```python
from build123d import *

# Parameters (mm, degrees)
SKETCH1_W           = 30
SKETCH1_H           = 12.2
BOSS_EXTRUDE1_DEPTH = 30
SKETCH2_W           = 26
SKETCH2_H           = 4.3
CUT_EXTRUDE1_DEPTH  = 26
SKETCH3_W           = 30
SKETCH3_H           = 30
BOSS_EXTRUDE2_DEPTH = 26
SKETCH4_W           = 17.8
SKETCH4_H           = 17.78
CUT_EXTRUDE2_DEPTH  = 26
SKETCH6_W           = 4.42
SKETCH6_H           = 26
CUT_EXTRUDE3_DEPTH  = 17.8
SKETCH9_W           = 4.3
SKETCH9_H           = 26
CUT_EXTRUDE4_DEPTH  = 17.8


with BuildPart() as part:
    # Sketch1 → Boss-Extrude1 (new body)
    with BuildSketch(Plane.XY):
        with Locations((-26.249929658, 18.197752809)):
            Rectangle(SKETCH1_W, SKETCH1_H)
    extrude(amount=BOSS_EXTRUDE1_DEPTH)

    # Sketch2 → Cut-Extrude1 (cut)
    with BuildSketch(Plane(origin=(-11.249929658, 0, 0), x_dir=(0, 0, -1), z_dir=(1, 0, 0))):
        with Locations((-17, 18.197752809)):
            Rectangle(SKETCH2_W, SKETCH2_H)
    extrude(amount=-CUT_EXTRUDE1_DEPTH, mode=Mode.SUBTRACT)

    # Sketch3 → Boss-Extrude2 (add)
    with BuildSketch(Plane(origin=(0, 24.297752809, 0), x_dir=(1, 0, 0), z_dir=(0, 1, 0))):
        with Locations((-26.249929658, -15)):
            Rectangle(SKETCH3_W, SKETCH3_H)
    extrude(amount=BOSS_EXTRUDE2_DEPTH)

    # Sketch4 → Cut-Extrude2 (cut)
    with BuildSketch(Plane(origin=(0, 50.297752809, 0), x_dir=(1, 0, 0), z_dir=(0, 1, 0))):
        with Locations((-20.149929658, -21.11)):
            Rectangle(SKETCH4_W, SKETCH4_H)
    extrude(amount=-CUT_EXTRUDE2_DEPTH, mode=Mode.SUBTRACT)

    # Sketch6 → Cut-Extrude3 (cut)
    with BuildSketch(Plane(origin=(-11.249929658, 0, 0), x_dir=(0, 0, -1), z_dir=(1, 0, 0))):
        with Locations((-6.11, 37.297752809)):
            Rectangle(SKETCH6_W, SKETCH6_H)
    extrude(amount=-CUT_EXTRUDE3_DEPTH, mode=Mode.SUBTRACT)

    # Sketch9 → Cut-Extrude4 (cut)
    with BuildSketch(Plane.XY.offset(30)):
        with Locations((-35.149929658, 37.297752809)):
            Rectangle(SKETCH9_W, SKETCH9_H)
    extrude(amount=-CUT_EXTRUDE4_DEPTH, mode=Mode.SUBTRACT)


solid = part.part
```
Here's how the part is built. I have some questions about the finished solid (model axes, mm). A direction names the side the tool comes from. Coordinates: 2 decimals unless noted, no trailing zeros. Write each loop counter-clockwise with the first axis right and the second up, starting at its lowest first coordinate (ties: lowest second). Pieces come first, ordered by that corner, then holes. Notation, with made-up numbers: M 16.5,-38 L 55.5,-38 A27 cw 55.5,-11 Z; hole C 4.25,-4.5 d5. An arc over 180 degrees is marked long. Answer as CSV lines item,"result". Start each with the question number.
Q1. Suppose I cut it at A-A, the plane z = 9.5. List the corners of the cut face in (x, y) for me, then the cut area to 3 significant figures.
Q2. Will these pins go through, and if not, where does the flat tip stop? pin 1 Ø3.5 at (y, z) = (18.5, 23) entering from +X; pin 2 Ø5.5 at (x, y) = (-19.5, 34.5) entering from +Z; pin 3 Ø14 at (y, z) = (35.5, 24.5) entering from +X.
Q3. For faces 1 (the flat face through (-37.3, 37, 21)), 2 (the flat face through (-20, 37, 8.32)), 3 (the flat face through (-37.25, 18, 17)), which set-ups out of +Z, -Z, +X, -X, +Y, -Y let a thin tool reach every point of the face, with its end or its side?
Q4. If we mould it in two halves opening along Z, with no side actions, what happens to faces 4 (the flat face through (-20, 24.298, 6)), 5 (the flat face through (-20, 37, 12.22)), 6 (the flat face through (-35, 24.298, 21))? For each: pulls with the +Z half, pulls with the -Z half, needs draft (parallel to the pull), parting line crosses it, or undercut.
Q5. Suppose I cut it at B-B, the plane x = -19.25. List the corners of the cut face in (y, z) for me, then the cut area to 3 significant figures.
Q6. I need wall thicknesses on probe 1 along Y at (x, z) = (-31, 10); probe 2 along Y at (x, z) = (-21, 28.5); probe 3 along X at (y, z) = (35.5, 27.25). Which ranges of each line are inside material? Lowest first, please. Write a range as [from, to].
Q7. Suppose I cut it at C-C, the plane y = 46.5. List the corners of the cut face in (x, z) for me.
Q8. Suppose I cut it at D-D, the plane x = -35. List the corners of the cut face in (y, z) for me, then the cut area to 3 significant figures.
Entries:
1,outline,"M -41.25,12.1 L -11.25,12.1 L -11.25,16.05 L -37.25,16.05 L -37.25,20.35 L -11.25,20.35 L -11.25,50.3 L -41.25,50.3 Z"
1,area,"1,030 mm²"
2,pin 1,"stops at x = -37.25"
2,pin 2,"stops at z = 12.22"
2,pin 3,"stops at x = -29.05"
3,face 1,"+Z, +Y"
3,face 2,"+X, +Y"
3,face 3,"+Z, +X"
4,face 4,"undercut"
4,face 5,"pulls with the +Z half"
4,face 6,"needs draft"
5,outline,"M 12.1,0 L 50.3,0 L 50.3,3.9 L 24.3,3.9 L 24.3,8.32 L 50.3,8.32 L 50.3,12.22 L 24.3,12.22 L 24.3,30 L 20.35,30 L 20.35,4 L 16.05,4 L 16.05,30 L 12.1,30 Z"
5,area,"457 mm²"
6,probe 1,"y = [12.1, 16.05], [20.35, 50.3]"
6,probe 2,"y = [12.1, 16.05], [20.35, 24.3]"
6,probe 3,"x = [-41.25, -37.3], [-33, -29.05]"
7,outline,"M -41.25,0 L -11.25,0 L -11.25,3.9 L -29.05,3.9 L -29.05,8.32 L -11.25,8.32 L -11.25,12.22 L -29.05,12.22 L -29.05,30 L -33,30 L -33,12.2 L -37.3,12.2 L -37.3,30 L -41.25,30 Z"
8,outline,"M 12.1,0 L 50.3,0 L 50.3,12.2 L 24.3,12.2 L 24.3,30 L 20.35,30 L 20.35,4 L 16.05,4 L 16.05,30 L 12.1,30 Z"
8,area,"571 mm²"
